from build123d import *

# Parameters (mm, degrees)
SKETCH1_R                = 24
SKETCH1_R_2              = 18
BOSS_EXTRUDE1_DEPTH      = 2
BOSS_EXTRUDE2_DEPTH      = 1
BOSS_EXTRUDE2_DEPTH_BACK = 1
BOSS_EXTRUDE3_DEPTH      = 1
BOSS_EXTRUDE3_DEPTH_BACK = 1
SKETCH5_R                = 1
BOSS_EXTRUDE4_DEPTH      = 4


with BuildPart() as part:
    # Sketch1 → Boss-Extrude1 (new body)
    with BuildSketch(Plane(origin=(0, 0, 0), x_dir=(1, 0, 0), z_dir=(0, 1, 0))):
        Circle(SKETCH1_R)
        Circle(SKETCH1_R_2, mode=Mode.SUBTRACT)
    extrude(amount=BOSS_EXTRUDE1_DEPTH)

    # Sketch3 → Boss-Extrude2 (add, two sides)
    with BuildSketch(Plane.XY) as boss_extrude2_sk:
        Polygon((24, 2), (21.979868871, 7), (10, 5.529057061), (10, 3.529057061), (18, 2), align=None)
        Polygon((-10, 3.529057061), (-18, 2), (-24, 2), (-21.979868871, 7), (-10, 5.529057061), align=None)
    extrude(amount=BOSS_EXTRUDE2_DEPTH)
    extrude(boss_extrude2_sk.sketch, amount=-BOSS_EXTRUDE2_DEPTH_BACK)

    # Sketch4 → Boss-Extrude3 (add, two sides)
    with BuildSketch(Plane(origin=(0, 0, 0), x_dir=(0, 0, -1), z_dir=(1, 0, 0))) as boss_extrude3_sk:
        Polygon((24, 2), (21.979868871, 7), (10, 5.529057061), (10, 3.529057061), (18, 2), align=None)
        Polygon((-10, 3.529057061), (-18, 2), (-24, 2), (-21.979868871, 7), (-10, 5.529057061), align=None)
    extrude(amount=BOSS_EXTRUDE3_DEPTH)
    extrude(boss_extrude3_sk.sketch, amount=-BOSS_EXTRUDE3_DEPTH_BACK)

    # Sketch5 → Boss-Extrude4 (add)
    with BuildSketch(Plane.XZ):
        with Locations((21, 0)):
            Circle(SKETCH5_R)
        with Locations((0, 21)):
            Circle(SKETCH5_R)
        with Locations((-21, 0)):
            Circle(SKETCH5_R)
        with Locations((0, -21)):
            Circle(SKETCH5_R)
    extrude(amount=BOSS_EXTRUDE4_DEPTH)


solid = part.part
Source: CAD feature listing. Evaluate the final solid. Frame: model axes, mm. A direction names the side the tool comes from. Round coordinates to 2 decimals unless told otherwise and drop trailing zeros. Loops run counter-clockwise (first coordinate to the right, second up) from the corner with the lowest first, then second, coordinate; pieces in that order, holes last. Notation, with made-up numbers: (44, -17) -> (95, -17) arc R6 ccw to (95, -8) -> close; hole circle Ø7 at (67.5, -34.75). An arc over 180 degrees is marked (long way). Answer as a JSON object with one key per item and string values. Group by question number.
Q1. Contact query for flat-ended pins moving along their axis: P1, Ø1.5, axis at x = 17, y = -0.5, coming from the -Z side; P2, Ø1.5, axis at x = 8.5, y = 0.5, coming from the -Z side; P3, Ø4, axis at x = -13.5, y = 5.5, coming from the -Z side; P4, Ø12, axis at x = -8, z = -8.5, coming from the +Y side. Output: stop coordinate, or through.
Q2. Section query A-A (z = -5). Output: boundary loops of the cut face in (x, y).
Q3. Ray query, line 1 (X direction, y = 0.75, z = 0); line 2 (Y direction, x = 18.5, z = -3). Return the intervals inside material, ascending. Write a range as from..to.
Q4. Section query C-C (x = -5). Output: boundary loops of the cut face in (y, z), plus the area to 3 significant figures.
Q5. Section query D-D (y = -3.25). Output: boundary loops of the cut face in (x, z).
Q6. Access query for faces 4 (the flat face through (1, 5, 17)), 5 (the flat face through (16.074, 6.275, 0.014)), 6 (the flat face through (-10, 5, 0)). Directions: +Z, -Z, +X, -X, +Y, -Y. A direction counts if a zero-diameter tool reaches every point of the face in a straight line with its end or side. Return the directions, or none.
Q7. Mould query, pull axis Z, two halves, no side actions, for faces 1 (the flat face through (23, 4.47, 0.01)), 2 (the cylindrical face through (-23.977, 0.986, -1.055)), 3 (the cylindrical face through (0, -2, -22)). Classes: pulls with the +Z half, pulls with the -Z half, needs draft (parallel to the pull), parting line crosses it, or undercut.
Q8. Section query B-B (x = 14.5). Output: boundary loops of the cut face in (y, z).
Completed:
{
 "1": {"P1": "z = -17.48", "P2": "z = -22.71", "P3": "z = -1", "P4": "through"},
 "2": {"outline": "(-23.47, 0) -> (-17.29, 0) -> (-17.29, 2) -> (-23.47, 2) -> close; (17.29, 0) -> (23.47, 0) -> (23.47, 2) -> (17.29, 2) -> close"},
 "3": {"line 1": "-24..-18, 18..24", "line 2": "0..2"},
 "4": {"outline": "(0, -23.47) -> (2, -23.47) -> (2, -17.29) -> (0, -17.29) -> close; (0, 17.29) -> (2, 17.29) -> (2, 23.47) -> (0, 23.47) -> close", "area": "24.7 mm²"},
 "5": {"outline": "circle Ø2 at (-21, 0); circle Ø2 at (0, -21); circle Ø2 at (0, 21); circle Ø2 at (21, 0)"},
 "6": {"face 4": "+Z, -Z, +X, +Y", "face 5": "+Z, -Z, +Y", "face 6": "+Z, -Z, +Y, -Y"},
 "7": {"face 1": "needs draft", "face 2": "parting line crosses it", "face 3": "undercut"},
 "8": {"outline": "(0, -19.12) -> (2, -19.12) -> (2, -10.67) -> (0, -10.67) -> close; (0, 10.67) -> (2, 10.67) -> (2, 19.12) -> (0, 19.12) -> close; (2.67, -1) -> (6.08, -1) -> (6.08, 1) -> (2.67, 1) -> close"}
}
